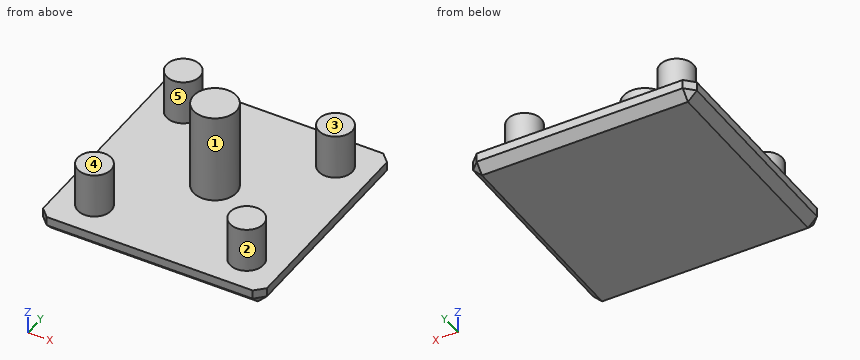
```python
from build123d import *

# Parameters (mm, degrees)
F0_W     = 25
F0_H     = 25
F1_DEPTH = 2
F2_R     = 2.4
F3_DEPTH = 10
F4_R     = 1.875
F5_DEPTH = 5
F6_SIZE  = 1


with BuildPart() as f1:
    # F0 (on Top) → F1 (new body)
    with BuildSketch(Plane.XY):
        Rectangle(F0_W, F0_H)
    extrude(amount=F1_DEPTH)

    # F2 (on face) → F3 (join)
    with BuildSketch(Plane.XY.offset(2)):
        Circle(F2_R)
    extrude(amount=F3_DEPTH)

    # F4 (on face) → F5 (join)
    with BuildSketch(Plane.XY.offset(2)):
        with Locations((-8.5, 8.5)):
            Circle(F4_R)
        with Locations((8.5, 8.5)):
            Circle(F4_R)
        with Locations((8.5, -8.5)):
            Circle(F4_R)
        with Locations((-8.5, -8.5)):
            Circle(F4_R)
    extrude(amount=F5_DEPTH)

    # F6
    f6_edges = [f1.edges().sort_by_distance(p)[0] for p in [
        (0, -12.5, 0),
        (12.5, 0, 0),
        (0, 12.5, 0),
        (-12.5, 0, 0),
        (-12.5, -12.5, 1),
        (12.5, -12.5, 1),
        (12.5, 12.5, 1),
        (-12.5, 12.5, 1),
    ]]
    chamfer(f6_edges, length=F6_SIZE)


solid = f1.part
```
Build history of the part. All positions in model axes, mm. Face numbers are marked on the shaded views. A direction names the side the tool comes from. Round coordinates to 2 decimals unless told otherwise and drop trailing zeros. Loops run counter-clockwise (first coordinate to the right, second up) from the corner with the lowest first, then second, coordinate; pieces in that order, holes last.
Item 1: Drill centre lines: line 1 along Z through (x, y) = (-10.25, 4.75); line 2 along Z through (x, y) = (8.75, 10); line 3 along X through (y, z) = (8.75, 2.25). Where is each one in solid material? Low to high.
Item 2: Pin check, flat tips, straight feed: P1, Ø4, axis at x = 6.5, y = -6.5, coming from the +Z side; P2, Ø4, axis at y = 3.5, z = 6, coming from the +X side; P3, Ø3, axis at x = 0.5, y = 3.5, coming from the +Z side; P4, Ø3, axis at x = -2.5, z = 8, coming from the -Y side. Stop position of each tip, or through.
Item 3: Saw through at B-B (x = 0). List the corners of the cut face in (y, z).
Item 4: Saw through at A-A (z = 4.25). List the corners of the cut face in (x, y) (3 decimals).
Item 5: Which spindle directions (+Z, -Z, +X, -X, +Y, -Y) get a long thin tool onto all of the face, cutting with end or side? Do the marked faces 4 and 5. Say none if no direction does.
Item 6: Two-plate mould, pull along X, no slides. Class the marked faces 1, 2 and 3: released by +X, released by -X, zero draft, split by the parting line, or undercut.
Item 7: Saw through at C-C (y = -8.5). List the corners of the cut face in (x, z) (3 decimals), then the cut area to 3 significant figures.
Worked answers:
1. line 1: z = 0 to 2
1. line 2: z = 0 to 7
1. line 3: x = -10.36 to -6.64, 6.64 to 10.36
2. P1: stops at z = 7
2. P2: stops at x = 1.87
2. P3: stops at z = 12
2. P4: stops at y = -2.18
3. outline: (-12.5, 1) - (-11.5, 0) - (11.5, 0) - (12.5, 1) - (12.5, 2) - (2.4, 2) - (2.4, 12) - (-2.4, 12) - (-2.4, 2) - (-12.5, 2) - close
4. outline: circle Ø3.75 at (-8.5, -8.5); circle Ø3.75 at (-8.5, 8.5); circle Ø4.8 at (0, 0); circle Ø3.75 at (8.5, -8.5); circle Ø3.75 at (8.5, 8.5)
5. face 4: +Z, +X, -X, +Y, -Y
5. face 5: +Z
6. face 1: split by the parting line
6. face 2: undercut
6. face 3: zero draft
7. outline: (-12.5, 1) - (-11.5, 0) - (11.5, 0) - (12.5, 1) - (12.5, 2) - (10.375, 2) - (10.375, 7) - (6.625, 7) - (6.625, 2) - (-6.625, 2) - (-6.625, 7) - (-10.375, 7) - (-10.375, 2) - (-12.5, 2) - close
7. area: 86.5 mm2
